Could you check a few things on this model? Use its own coordinates, in mm. Face numbers are marked on the shaded views. A direction names the side the tool comes from. Coordinates: 2 decimals unless noted, no trailing zeros. Loops run counter-clockwise (first coordinate to the right, second up) from the corner with the lowest first, then second, coordinate; pieces in that order, holes last. Notation, with made-up numbers: M 19,50.5 L 69,50.5 A17 cw 69,76.5 Z; hole C -36,-11 d10. An arc over 180 degrees is marked long. Write each question's results on one line, items separated by ' | '.
```python
from build123d import *

# Parameters (mm, degrees)
SKETCH2_R                = 2.25
BOSS_EXTRUDE2_DEPTH      = 5
BOSS_EXTRUDE3_DEPTH      = 85
SKETCH2_2_R              = 2.25
CUT_EXTRUDE1_DEPTH       = 5
SKETCH9_W                = 20
SKETCH9_H                = 85
BOSS_EXTRUDE6_DEPTH      = 21.72
BOSS_EXTRUDE7_DEPTH      = 75
BOSS_EXTRUDE7_DEPTH_BACK = 20
FILLET2_R                = 15
SKETCH12_W               = 40
SKETCH12_H               = 246
CUT_EXTRUDE2_DEPTH       = 75
CHAMFER2_SIZE            = 15


with BuildPart() as part:
    # Sketch2 → Boss-Extrude2 (new body)
    with BuildSketch(Plane(origin=(0, 0, 0), x_dir=(0, 1, 0), z_dir=(0, 0, 1))):
        with BuildLine():
            Line((3.872983346, 1), (16, 1))
            Line((16, 1), (16, -1))
            Line((16, -1), (3.872983346, -1))
            ThreePointArc((3.872983346, -1), (-4, 0), (3.872983346, 1))
        make_face()
        with Locations(Location((0, 0, 0), (0, 0, 270))):
            Circle(SKETCH2_R, mode=Mode.SUBTRACT)
    extrude(amount=BOSS_EXTRUDE2_DEPTH)

    # Sketch4 → Boss-Extrude3 (add)
    with BuildSketch(Plane(origin=(0, 0, 0), x_dir=(1, 0, 0), z_dir=(0, 0, -1))):
        with BuildLine():
            Line((-2.5, 5.5), (2.5, 5.5))
            ThreePointArc((2.5, 5.5), (6.035533906, 4.035533906), (7.5, 0.5))
            Line((7.5, 0.5), (7.5, -19.5))
            Line((7.5, -19.5), (-7.5, -19.5))
            Line((-7.5, -19.5), (-7.5, 0.5))
            ThreePointArc((-7.5, 0.5), (-6.035533906, 4.035533906), (-2.5, 5.5))
        make_face()
    extrude(amount=-BOSS_EXTRUDE3_DEPTH)

    # Sketch2<2> → Cut-Extrude1 (cut)
    with BuildSketch(Plane(origin=(0, 0, 0), x_dir=(0, 1, 0), z_dir=(0, 0, 1))):
        with BuildLine():
            Line((3.872983346, 1), (16, 1))
            Line((16, 1), (16, -1))
            Line((16, -1), (3.872983346, -1))
            ThreePointArc((3.872983346, -1), (-4, 0), (3.872983346, 1))
        make_face()
        with Locations(Location((0, 0, 0), (0, 0, 270))):
            Circle(SKETCH2_2_R, mode=Mode.SUBTRACT)
    cut_extrude1 = extrude(amount=CUT_EXTRUDE1_DEPTH, mode=Mode.SUBTRACT)

    # Mirror1: Cut-Extrude1 across plane
    add(cut_extrude1.mirror(Plane.XY.offset(42.5)), mode=Mode.SUBTRACT)

    # Sketch9 → Boss-Extrude6 (add)
    with BuildSketch(Plane.YZ.offset(7.5)):
        with Locations((9.5, 42.5)):
            Rectangle(SKETCH9_W, SKETCH9_H)
    extrude(amount=BOSS_EXTRUDE6_DEPTH)

    # Sketch11 → Boss-Extrude7 (add, two sides: drawn at the far end of the back side and taken through both)
    with BuildSketch(Plane(origin=(0, 19.5, 0), x_dir=(-1, 0, 0), z_dir=(0, 1, 0)).offset(-BOSS_EXTRUDE7_DEPTH_BACK)):
        Polygon((-27.22, 0), (-14.22, 0), (-14.22, -82.5), (-29.22, -82.5), (-29.22, 167.5), (-14.22, 167.5), (-14.22, 85), (-27.22, 85), align=None)
    extrude(amount=BOSS_EXTRUDE7_DEPTH + BOSS_EXTRUDE7_DEPTH_BACK)

    # Fillet2
    fillet2_edges = [part.edges().sort_by_distance(p)[0] for p in [
        (29.22, -0.5, 42.5),
    ]]
    fillet(fillet2_edges, radius=FILLET2_R)

    # Sketch12 → Cut-Extrude2 (cut)
    with BuildSketch(Plane(origin=(0, 94.5, 0), x_dir=(-1, 0, 0), z_dir=(0, 1, 0))):
        with Locations((-7.22, 42.5)):
            Rectangle(SKETCH12_W, SKETCH12_H)
    extrude(amount=-CUT_EXTRUDE2_DEPTH, mode=Mode.SUBTRACT)

    # Chamfer2
    chamfer2_edges = [part.edges().sort_by_distance(p)[0] for p in [
        (14.22, 94.5, 166.5),
    ]]
    chamfer(chamfer2_edges, length=CHAMFER2_SIZE - 0.0001)  # a hair under: the kernel refuses the full size


solid = part.part
```
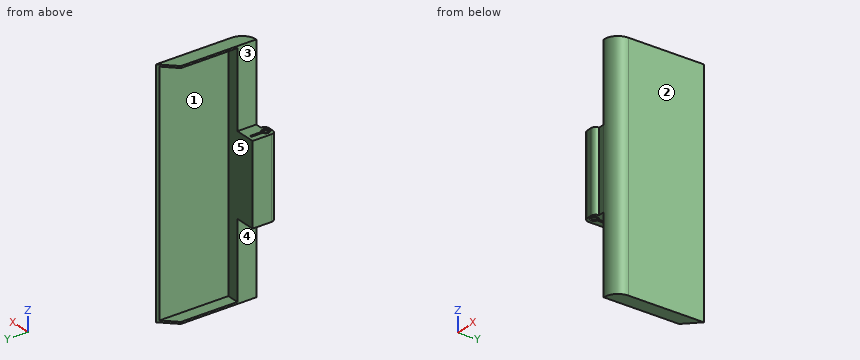
(1) If we mould it in two halves opening along Z, with no side actions, what happens to the marked faces 4 and 5? For each: released by +Z, released by -Z, zero draft, split by the parting line, or undercut.
Reported:
face 4: zero draft | face 5: undercut
(2) Will these pins go through, and if not, where does the flat tip stop? P1, Ø6.5, axis at x = 3, y = 11.5, coming from the -Z side; P2, Ø10.5, axis at x = 3.5, z = 27, coming from the +Y side; P3, Ø5, axis at x = 0, y = 0, coming from the +Z side.
Reported:
P1: stops at z = 0 | P2: stops at y = 19.5 | P3: stops at z = 85
(3) Imagine slicing it at A-A, the plane y = 54. List the corners of the cut face in (x, z) for me, and give its area (3 significant figures).
Reported:
outline: M 14.22,-82.5 L 29.22,-82.5 L 29.22,167.5 L 14.22,167.5 L 14.22,165.5 L 27.22,165.5 L 27.22,-80.5 L 14.22,-80.5 Z | area: 552 mm2
(4) Imagine slicing it at C-C, the plane x = 11. List the corners of the cut face in (y, z) for me, and give its area (3 significant figures).
Reported:
outline: M -0.5,0 L 19.5,0 L 19.5,85 L -0.5,85 Z | area: 1,700 mm2
(5) Imagine slicing it at D-D, the plane y = 87.5. List the corners of the cut face in (x, z) for me, and give its area (3 significant figures).
Reported:
outline: M 22.22,-82.5 L 29.22,-82.5 L 29.22,167.5 L 22.22,167.5 L 22.22,165.5 L 27.22,165.5 L 27.22,-80.5 L 22.22,-80.5 Z | area: 520 mm2
(6) Which directions (+Z, -Z, +X, -X, +Y, -Y) give clear straight access to the entire face, cutting with the end or side of a thin tool? Please do the marked faces 1, 2 and 3.
Reported:
face 1: -X, +Y | face 2: +Z, -Z, +X, +Y, -Y | face 3: +Z, -X, +Y, -Y
(7) Please list where these lines run through material, in increasing order: probe 1 along Y at (x, z) = (0, 1.9); probe 2 along Z at (x, y) = (14.5, 56.5); probe 3 along X at (y, z) = (34, -56). Write a range as from..to.
Reported:
probe 1: y = -5.5..-4, -2.25..2.25, 16..19.5 | probe 2: z = -82.5..-80.5, 165.5..167.5 | probe 3: x = 27.22..29.22
